Geometry: final body of the model. Coordinates: model frame, mm. Round coordinates to 2 decimals unless told otherwise and drop trailing zeros. Loops run counter-clockwise (first coordinate to the right, second up) from the corner with the lowest first, then second, coordinate; pieces in that order, holes last. Notation, with made-up numbers: M -28.5,-19.75 L 15.5,-19.75 A19 ccw 15.5,5.25 Z; hole C 89,-2 d6. An arc over 180 degrees is marked long. Write each question's results on one line, items separated by ' | '.
```python
from build123d import *

# Parameters (mm, degrees)
F0_W     = 62.9
F0_H     = 57.8
F1_DEPTH = 28
F2_R     = 7
F4_DEPTH = 5


with BuildPart() as f1:
    # F0 (on Front) → F1 (new body)
    with BuildSketch(Plane.XZ):
        with Locations((31.45, 28.9)):
            Rectangle(F0_W, F0_H)
    extrude(amount=F1_DEPTH)

    # F2
    f2_edges = [f1.edges().sort_by_distance(p)[0] for p in [
        (0, -28, 28.9),
        (0, 0, 28.9),
        (62.9, -28, 28.9),
        (62.9, 0, 28.9),
    ]]
    fillet(f2_edges, radius=F2_R)

    # F3 (on face) → F4 (join)
    with BuildSketch(Plane(origin=(0, 0, 0), x_dir=(1, 0, 0), z_dir=(0, 0, -1))):
        with BuildLine():
            Line((55.9, 14), (42.9, 14))
            ThreePointArc((42.9, 14), (35.9, 7), (42.9, 0))
            Line((42.9, 0), (55.9, 0))
            ThreePointArc((55.9, 0), (62.9, 7), (55.9, 14))
        make_face()
    extrude(amount=F4_DEPTH)


solid = f1.part
```
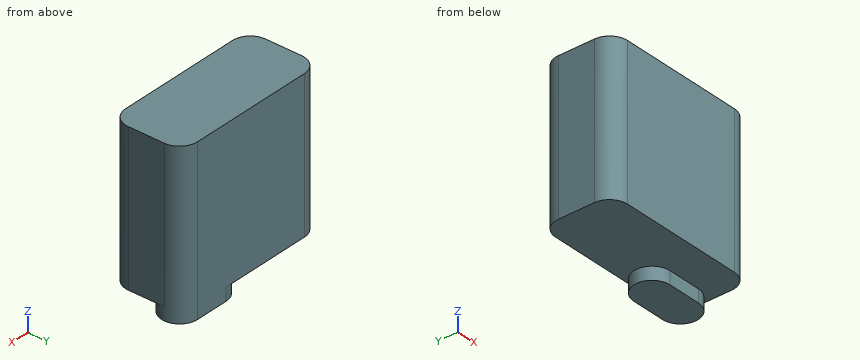
1. Ray query, probe 1 along Z at (x, y) = (18.5, -7.25); probe 2 along X at (y, z) = (-22, 13); probe 3 along X at (y, z) = (-2.25, -1.5). Return the intervals inside material, ascending.
Answer key:
probe 1: z = 0 to 57.8 | probe 2: x = 0.07 to 62.83 | probe 3: x = 37.76 to 61.04
2. Section C-C (y = -16). Output: boundary loops of the cut face in (x, z).
Answer key:
outline: M 0,0 L 62.9,0 L 62.9,57.8 L 0,57.8 Z
3. Section B-B (x = 40). Output: boundary loops of the cut face in (y, z).
Answer key:
outline: M -28,0 L -13.37,0 L -13.37,-5 L -0.63,-5 L -0.63,0 L 0,0 L 0,57.8 L -28,57.8 Z
4. Section A-A (z = 32.5). Output: boundary loops of the cut face in (x, y).
Answer key:
outline: M 0,-21 A7 ccw 7,-28 L 55.9,-28 A7 ccw 62.9,-21 L 62.9,-7 A7 ccw 55.9,0 L 7,0 A7 ccw 0,-7 Z
5. Pin query (flat end, axial travel): P1, Ø1, axis at x = 55, y = -24, coming from the -Z side; P2, Ø4, axis at x = 48.5, z = -3, coming from the -Y side. Return the tip coordinate at first contact, or that it passes through.
Answer key:
P1: stops at z = 0 | P2: stops at y = -14
6. Section D-D (x = 9.5). Output: boundary loops of the cut face in (y, z), then the cut area to 3 significant figures.
Answer key:
outline: M -28,0 L 0,0 L 0,57.8 L -28,57.8 Z | area: 1,620 mm²
